```python
from build123d import *

# Parameters (mm, degrees)
SKETCH1_W                 = 100
SKETCH1_H                 = 10
BOSS_EXTRUDE1_DEPTH       = 100
SKETCH2_R                 = 10
SKETCH2_R_2               = 5
BOSS_EXTRUDE2_DEPTH       = 10
MIRROR2_COPY_1_SKETCH_R   = 10
MIRROR2_COPY_1_SKETCH_R_2 = 5
MIRROR2_COPY_1_DEPTH      = 10
SKETCH3_W                 = 175
SKETCH3_H                 = 55
SKETCH3_W_2               = 170
SKETCH3_H_2               = 50
BOSS_EXTRUDE5_DEPTH       = 50


with BuildPart() as part:
    # Sketch1 → Boss-Extrude1 (new body, symmetric)
    with BuildSketch(Plane(origin=(0, 0, 0), x_dir=(0, 0, -1), z_dir=(1, 0, 0))):
        Rectangle(SKETCH1_W, SKETCH1_H)
    extrude(amount=BOSS_EXTRUDE1_DEPTH, both=True)

    # Sketch2 → Boss-Extrude2 (add)
    with BuildSketch(Plane(origin=(100, 0, 0), x_dir=(0, 0, -1), z_dir=(1, 0, 0))):
        with Locations((-40, 15)):
            Circle(SKETCH2_R)
        with Locations((-40, 15)):
            Circle(SKETCH2_R_2, mode=Mode.SUBTRACT)
        with BuildLine():
            ThreePointArc((-40, 5), (-47.071067812, 7.928932188), (-50, 15))
            Line((-50, 15), (-50, 5))
            Line((-50, 5), (-40, 5))
        make_face()
        with BuildLine():
            Line((-30, 5), (-30, 15))
            ThreePointArc((-30, 15), (-32.928932188, 7.928932188), (-40, 5))
            Line((-40, 5), (-30, 5))
        make_face()
    boss_extrude2 = extrude(amount=-BOSS_EXTRUDE2_DEPTH)

    # Mirror1: Boss-Extrude2 across plane
    add(boss_extrude2.mirror(Plane.XY))

    # Mirror2: Boss-Extrude2 across plane
    add(boss_extrude2.mirror(Plane(origin=(0, 0, 0), x_dir=(0, 0, 1), z_dir=(1, 0, 0))))

    # Mirror2 copy 1 sketch → Mirror2 copy 1 (add)
    with BuildSketch(Plane.ZY.offset(100)):
        with Locations((-40, 15)):
            Circle(MIRROR2_COPY_1_SKETCH_R)
        with Locations((-40, 15)):
            Circle(MIRROR2_COPY_1_SKETCH_R_2, mode=Mode.SUBTRACT)
        with BuildLine():
            ThreePointArc((-40, 5), (-47.071067812, 7.928932188), (-50, 15))
            Line((-50, 15), (-50, 5))
            Line((-50, 5), (-40, 5))
        make_face()
        with BuildLine():
            Line((-30, 5), (-30, 15))
            ThreePointArc((-30, 15), (-32.928932188, 7.928932188), (-40, 5))
            Line((-40, 5), (-30, 5))
        make_face()
    extrude(amount=-MIRROR2_COPY_1_DEPTH)

    # Sketch3 → Boss-Extrude5 (add)
    with BuildSketch(Plane(origin=(0, 5, 0), x_dir=(1, 0, 0), z_dir=(0, 1, 0))):
        Rectangle(SKETCH3_W, SKETCH3_H)
        Rectangle(SKETCH3_W_2, SKETCH3_H_2, mode=Mode.SUBTRACT)
    extrude(amount=BOSS_EXTRUDE5_DEPTH)


solid = part.part
```
Check sheet for the modelled part. Datum: model origin and axes. Units: mm. A direction names the side the tool comes from. Give positions to 0.01 mm unless a question says otherwise; leave off trailing zeros. Order: outer loops, then holes, each group sorted by start corner. A loop starts at its lowest first (then second) coordinate and runs counter-clockwise, first axis right, second up. Notation, with made-up numbers: (68, 23.25) -> (84, 23.25) arc R18 cw to (84, 36.25) -> close; hole circle Ø1 at (71.5, 20.25). An arc over 180 degrees is marked (long way). Use CSV: the item, a comma, the result in double quotes. Start each with the question number.
1) Sectioned sample at B-B, the plane z = -40. Record the boundary of the cut face in (x, y).
2) Mould release check, pull along Z, two halves, no side actions. Record for faces 5 (the face through (-1, 30, 27.5)), 6 (the face through (-95, 12, 44)), 7 (the face through (1, -5, 1)): released by +Z, released by -Z, zero draft, split by the parting line, or undercut.
3) Set-up check for faces 1 (the face through (-1, 30, 25)), 2 (the face through (87.5, 30, 0)), 3 (the face through (95, 10, 30)), 4 (the face through (90, 13, -45)): record each of +Z, -Z, +X, -X, +Y, -Y from which the full face is reachable in a straight line by a thin tool's end or side.
4) Go/stop test with flat-tipped pins: P1, Ø5, axis at x = -5, y = 9, coming from the +Z side; P2, Ø12, axis at y = 46, z = -25, coming from the +X side; P3, Ø25, axis at x = 9, z = -3, coming from the +Y side. Record where each tip stops, or that it passes through.
5) Sectioned sample at A-A, the plane y = 23. Record the boundary of the cut face in (x, z).
6) Material ranges on line 1 (X direction, y = 43, z = 14.5); line 2 (Y direction, x = -92, z = 40); line 3 (X direction, y = 7, z = 42.5), recorded low to high. Write a range as from..to.
7) Sectioned sample at C-C, the plane x = 71. Record the boundary of the cut face in (y, z), plus the area to 3 significant figures.
8) Sectioned sample at D-D, the plane z = -2. Record the boundary of the cut face in (x, y), plus the area to 3 significant figures.
Recorded:
1,outline,"(-100, -5) -> (100, -5) -> (100, 10) -> (90, 10) -> (90, 5) -> (-90, 5) -> (-90, 10) -> (-100, 10) -> close; (-100, 20) -> (-90, 20) -> (-90, 25) -> (-100, 25) -> close; (90, 20) -> (100, 20) -> (100, 25) -> (90, 25) -> close"
2,face 5,"released by +Z"
2,face 6,"undercut"
2,face 7,"zero draft"
3,face 1,"+Y"
3,face 2,"+Z, -Z, +X, +Y"
3,face 3,"+X, -X, +Y"
3,face 4,"+Z, -Z, +Y"
4,P1,"z = 27.5"
4,P2,"x = 87.5"
4,P3,"y = 5"
5,outline,"(-100, -46) -> (-90, -46) -> (-90, -34) -> (-100, -34) -> close; (-100, 34) -> (-90, 34) -> (-90, 46) -> (-100, 46) -> close; (-87.5, -27.5) -> (87.5, -27.5) -> (87.5, 27.5) -> (-87.5, 27.5) -> close; (90, -46) -> (100, -46) -> (100, -34) -> (90, -34) -> close; (90, 34) -> (100, 34) -> (100, 46) -> (90, 46) -> close; hole (-85, -25) -> (85, -25) -> (85, 25) -> (-85, 25) -> close"
6,line 1,"-87.5..-85, 85..87.5"
6,line 2,"-5..10, 20..25"
6,line 3,"-100..-90, 90..100"
7,outline,"(-5, -50) -> (5, -50) -> (5, -27.5) -> (55, -27.5) -> (55, -25) -> (5, -25) -> (5, 25) -> (55, 25) -> (55, 27.5) -> (5, 27.5) -> (5, 50) -> (-5, 50) -> close"
7,area,"1,250 mm2"
8,outline,"(-100, -5) -> (100, -5) -> (100, 5) -> (87.5, 5) -> (87.5, 55) -> (85, 55) -> (85, 5) -> (-85, 5) -> (-85, 55) -> (-87.5, 55) -> (-87.5, 5) -> (-100, 5) -> close"
8,area,"2,250 mm2"
